Geometry: see drawing. Coordinates: mm, zero at the bounding-box minimum. Round coordinates to 2 decimals unless told otherwise and drop trailing zeros. Loops run counter-clockwise (first coordinate to the right, second up) from the corner with the lowest first, then second, coordinate; pieces in that order, holes last. Notation, with made-up numbers: M -1,21 L 52,21 A10 ccw 52,37 Z; hole C 2,66 d11. An arc over 180 degrees is marked long. Answer as a JSON object with one key per item and string values.
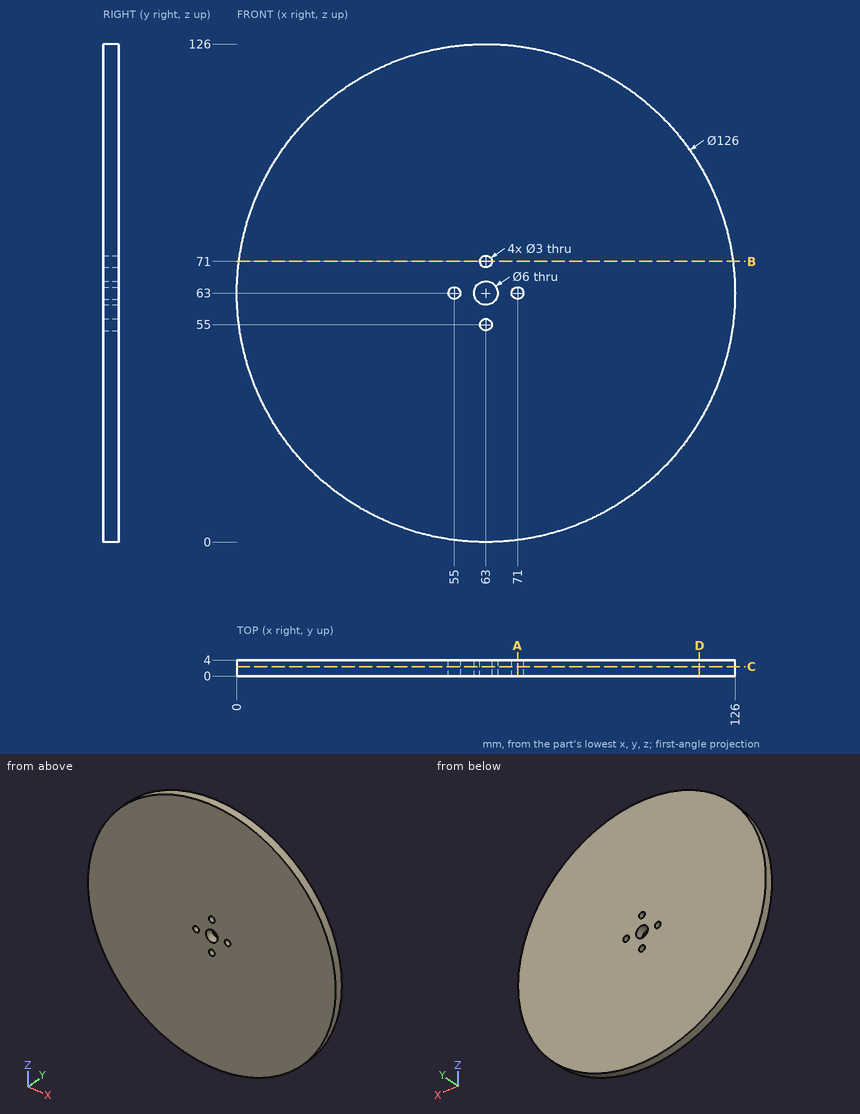
1) Section query A-A (x = 71). Return the cut outline in (y, z).
Results:
{"outline": "M 0,0.51 L 4,0.51 L 4,61.5 L 0,61.5 Z; M 0,64.5 L 4,64.5 L 4,125.49 L 0,125.49 Z"}
2) Pin query (flat end, axial travel): P1, Ø1.5, axis at x = 85, y = 1.5, coming from the -Z side. Return the tip coordinate at first contact, or that it passes through.
Results:
{"P1": "z = 3.69"}
3) Section query B-B (z = 71). Return the cut outline in (x, y), and give its area (3 significant figures).
Results:
{"outline": "M 0.51,0 L 61.5,0 L 61.5,4 L 0.51,4 Z; M 64.5,0 L 125.49,0 L 125.49,4 L 64.5,4 Z", "area": "488 mm2"}
4) Ray query, line 1 (X direction, y = 3, z = 63); line 2 (Z direction, x = 63.5, y = 3.65). Return the intervals inside material, ascending.
Results:
{"line 1": "0 to 53.5, 56.5 to 60, 66 to 69.5, 72.5 to 126", "line 2": "0 to 53.59, 56.41 to 60.04, 65.96 to 69.59, 72.41 to 126"}
5) Section query D-D (x = 117). Return the cut outline in (y, z), and give its area (3 significant figures).
Results:
{"outline": "M 0,30.55 L 4,30.55 L 4,95.45 L 0,95.45 Z", "area": "260 mm2"}
6) Section query C-C (y = 2.35). Return the cut outline in (x, z).
Results:
{"outline": "C 63,63 d126; hole C 55,63 d3; hole C 63,63 d6; hole C 63,55 d3; hole C 63,71 d3; hole C 71,63 d3"}
